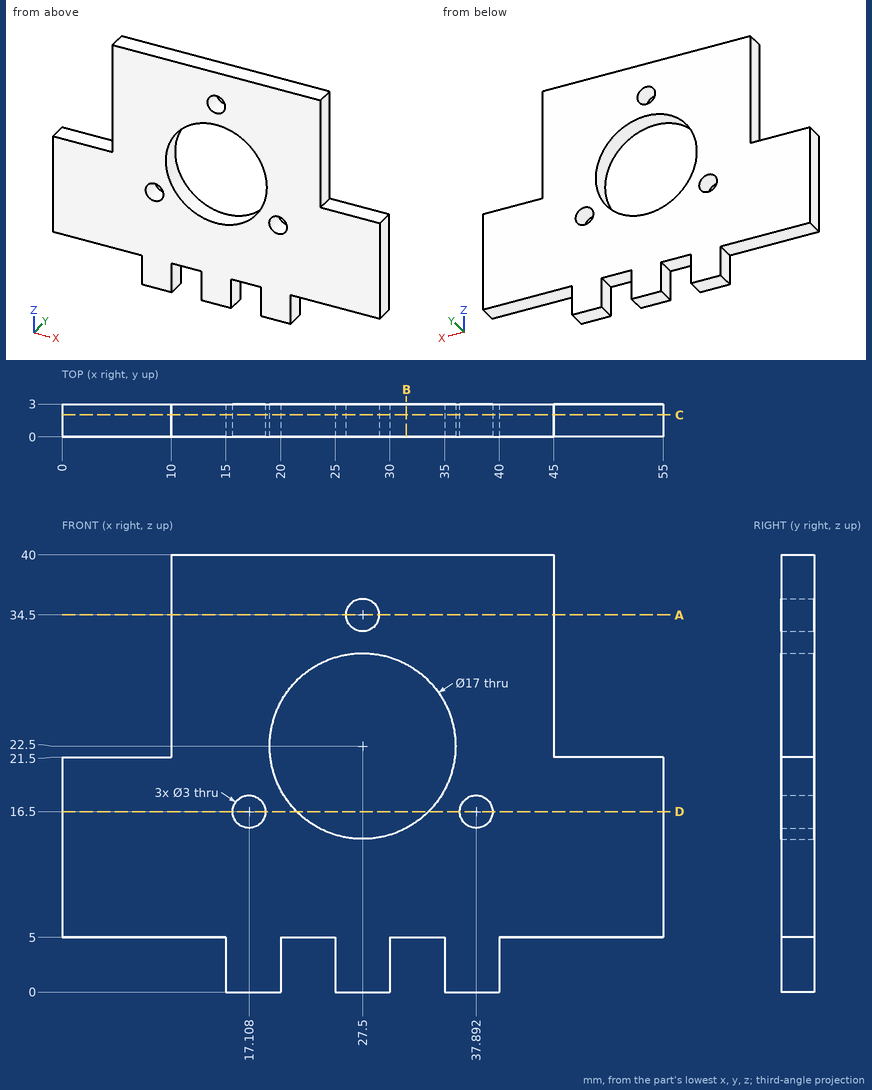
Geometry check sheet. Reference: drawing and pictorial views, mm from the part's lowest x, y, z. Give positions to 0.01 mm unless a question says otherwise; leave off trailing zeros. Order: outer loops, then holes, each group sorted by start corner. A loop starts at its lowest first (then second) coordinate and runs counter-clockwise, first axis right, second up. Notation, with made-up numbers: (-33, 48) - (15, 48) arc R26 ccw to (15, 71) - close; hole circle Ø6 at (32.25, 89). An arc over 180 degrees is marked (long way). Answer as CSV lines item,"result". Start each with the question number.
Item 1: Material ranges on L1, parallel to Z at x = 27.5, y = 1.05; L2, parallel to X at y = 2.3, z = 2; L3, parallel to X at y = 1.6, z = 16 (1 decimal), recorded low to high.
Item 2: Section check C-C, the plane y = 2. Record the boundary of the cut face in (x, z).
Item 3: Section check D-D, the plane z = 16.5. Record the boundary of the cut face in (x, y).
Item 4: Section check A-A, the plane z = 34.5. Record the boundary of the cut face in (x, y), plus the area to 3 significant figures.
Item 5: Gauge pin test, flat ends, axial feed: pin 1 (0.9 mm diameter, centred on x = 4.5, y = 2, fed in from -Z); pin 2 (1 mm diameter, centred on y = 1, z = 30, fed in from -X); pin 3 (1.5 mm diameter, centred on y = 1.5, z = 3.5, fed in from -X); pin 4 (15.5 mm diameter, centred on x = 27.5, z = 22.5, fed in from +Y). Record the tip position at first contact, or that the pin passes through.
Item 6: Section check B-B, the plane x = 31.5. Record the boundary of the cut face in (y, z).
Filled in:
1,L1,"0 to 14, 31 to 33, 36 to 40"
1,L2,"15 to 20, 25 to 30, 35 to 40"
1,L3,"0 to 15.7, 18.5 to 22, 33 to 36.5, 39.3 to 55"
2,outline,"(0, 5) - (15, 5) - (15, 0) - (20, 0) - (20, 5) - (25, 5) - (25, 0) - (30, 0) - (30, 5) - (35, 5) - (35, 0) - (40, 0) - (40, 5) - (55, 5) - (55, 21.5) - (45, 21.5) - (45, 40) - (10, 40) - (10, 21.5) - (0, 21.5) - close; hole circle Ø3 at (17.11, 16.5); hole circle Ø17 at (27.5, 22.5); hole circle Ø3 at (27.5, 34.5); hole circle Ø3 at (37.89, 16.5)"
3,outline,"(0, 0) - (15.61, 0) - (15.61, 3) - (0, 3) - close; (18.61, 0) - (21.48, 0) - (21.48, 3) - (18.61, 3) - close; (33.52, 0) - (36.39, 0) - (36.39, 3) - (33.52, 3) - close; (39.39, 0) - (55, 0) - (55, 3) - (39.39, 3) - close"
4,outline,"(10, 0) - (26, 0) - (26, 3) - (10, 3) - close; (29, 0) - (45, 0) - (45, 3) - (29, 3) - close"
4,area,"96.0 mm^2"
5,pin 1,"z = 5"
5,pin 2,"x = 10"
5,pin 3,"x = 15"
5,pin 4,"through"
6,outline,"(0, 5) - (3, 5) - (3, 15) - (0, 15) - close; (0, 30) - (3, 30) - (3, 40) - (0, 40) - close"
